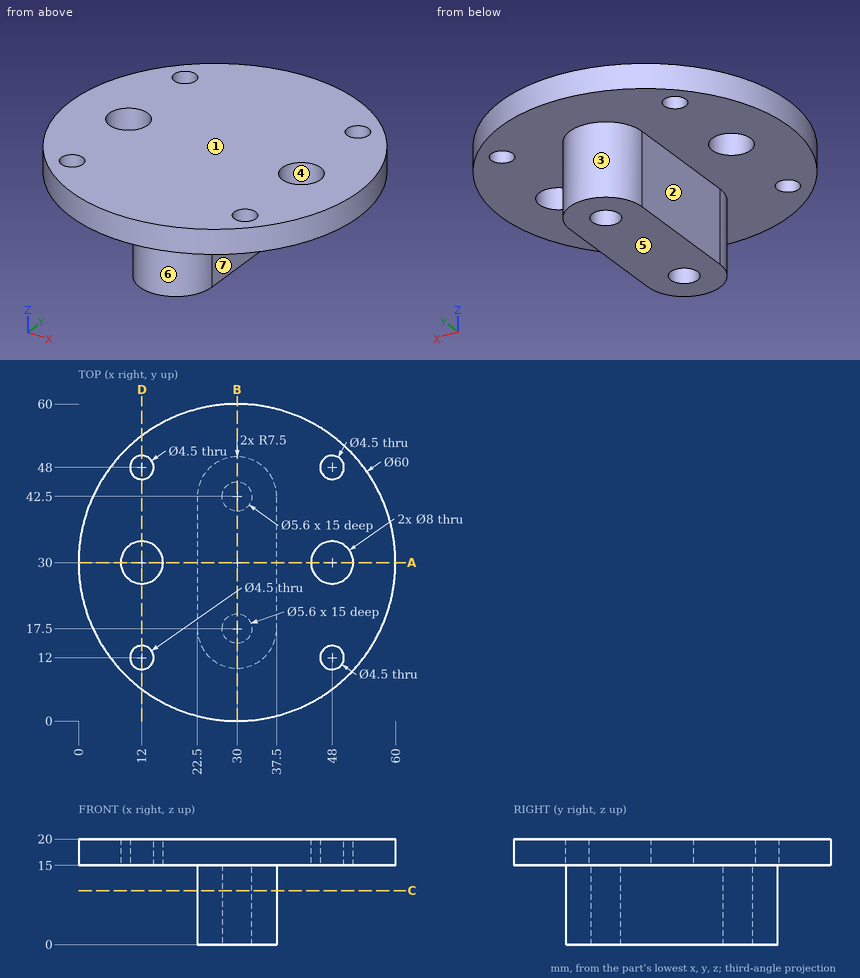
Could you check a few things on this drawing? It's one solid part, dimensions in mm from its lowest x, y, z. A direction names the side the tool comes from. Round coordinates to 2 decimals unless told otherwise and drop trailing zeros. Order: outer loops, then holes, each group sorted by start corner. A loop starts at its lowest first (then second) coordinate and runs counter-clockwise, first axis right, second up. Notation, with made-up numbers: M 32,64 L 56,64 A12 ccw 56,85 Z; hole C -8,-12 d8. An arc over 180 degrees is marked long. One line per item, written item: value.
(1) Which directions (+Z, -Z, +X, -X, +Y, -Y) give clear straight access to the entire face, cutting with the end or side of a thin tool? Please do the marked faces 5, 6 and 7.
Ans:
face 5: -Z, +X, -X, +Y, -Y
face 6: -Z, -Y
face 7: -Z, +X, +Y, -Y
(2) I'm going to push flat-ended pins straight in: P1, Ø1, axis at y = 22, z = 4, coming from the +X side; P2, Ø6, axis at x = 31.5, y = 44, coming from the -Z side; P3, Ø4.5, axis at y = 29.5, z = 8, coming from the -X side; P4, Ø4, axis at y = 27, z = 14, coming from the +X side. Where does each tip first touch, or does it pass through?
Ans:
P1: stops at x = 37.5
P2: stops at z = 0
P3: stops at x = 22.5
P4: stops at x = 59.97
(3) Imagine slicing it at B-B (x = 30). Write out the boundary of the cut face in (y, z).
Ans:
outline: M 0,15 L 10,15 L 10,0 L 14.7,0 L 14.7,15 L 20.3,15 L 20.3,0 L 39.7,0 L 39.7,15 L 45.3,15 L 45.3,0 L 50,0 L 50,15 L 60,15 L 60,20 L 0,20 Z
(4) Imagine slicing it at C-C (z = 10.25). Write out the boundary of the cut face in (x, y).
Ans:
outline: M 22.5,17.5 A7.5 ccw 37.5,17.5 L 37.5,42.5 A7.5 ccw 22.5,42.5 Z; hole C 30,17.5 d5.6; hole C 30,42.5 d5.6
(5) If we mould it in two halves opening along X, with no side actions, what happens to the marked faces 1, 2, 3 and 4? For each: released by +X, released by -X, zero draft, split by the parting line, or undercut.
Ans:
face 1: zero draft
face 2: released by -X
face 3: split by the parting line
face 4: undercut
(6) Imagine slicing it at A-A (y = 30). Write out the boundary of the cut face in (x, z), and give its area (3 significant figures).
Ans:
outline: M 0,15 L 8,15 L 8,20 L 0,20 Z; M 16,15 L 22.5,15 L 22.5,0 L 37.5,0 L 37.5,15 L 44,15 L 44,20 L 16,20 Z; M 52,15 L 60,15 L 60,20 L 52,20 Z
area: 445 mm^2
(7) Imagine slicing it at D-D (x = 12). Write out the boundary of the cut face in (y, z), and give its area (3 significant figures).
Ans:
outline: M 6,15 L 9.75,15 L 9.75,20 L 6,20 Z; M 14.25,15 L 26,15 L 26,20 L 14.25,20 Z; M 34,15 L 45.75,15 L 45.75,20 L 34,20 Z; M 50.25,15 L 54,15 L 54,20 L 50.25,20 Z
area: 155 mm^2
(8) I need wall thicknesses on line 1 along Y through (x, z) = (12, 18.9); line 2 along X through (y, z) = (46.5, 18.25); line 3 along Z through (x, y) = (48.5, 42). Which ranges of each line are inside material? Lowest first, please. Write a range as from..to.
Ans:
line 1: y = 6..9.75, 14.25..26, 34..45.75, 50.25..54
line 2: x = 4.95..10.32, 13.68..46.32, 49.68..55.05
line 3: z = 15..20
